from build123d import *

# Parameters (mm, degrees)
BOSS_EXTRUDE1_DEPTH      = 40
CHAMFER1_SIZE            = 25
SKETCH3_W                = 55
SKETCH3_H                = 30.849850196
CUT_EXTRUDE2_DEPTH       = 3
SKETCH5_R                = 1.75
CUT_EXTRUDE4_DEPTH       = 56.226805086
CUT_EXTRUDE3_DEPTH       = 38
SKETCH6_R                = 5.5
SKETCH6_R_2              = 3
BOSS_EXTRUDE2_DEPTH      = 5
CUT_EXTRUDE5_START       = -2
SKETCH7_R                = 3
CUT_EXTRUDE5_DEPTH       = 2
SKETCH9_R                = 3.75
CUT_EXTRUDE7_DEPTH       = 24
SKETCH10_W               = 80.05733418
SKETCH10_H               = 23.210803027
CUT_EXTRUDE8_DEPTH       = 27
BOSS_EXTRUDE3_REACH      = 57.227
BOSS_EXTRUDE3_END_RADIUS = 5.5
SKETCH13_W               = 5
SKETCH13_H               = 8
SKETCH14_W               = 8.301356979
SKETCH14_H               = 17.411858477
CUT_EXTRUDE9_DEPTH       = 38
SKETCH15_W               = 30
SKETCH15_H               = 2
BOSS_EXTRUDE4_DEPTH      = 10


with BuildPart() as part:
    # Sketch1 → Boss-Extrude1 (new body)
    with BuildSketch(Plane.XY):
        Polygon((-27.5, 0), (27.5, 0), (27.5, -15), (35, -10), (35, 0), (27.5, 10), (-27.5, 10), (-35, 0), (-35, -10), (-27.5, -15), align=None)
    extrude(amount=BOSS_EXTRUDE1_DEPTH)

    # Chamfer1
    # the kernel refuses this chamfer: 25 mm, written as the material it takes off along each edge
    with BuildSketch(Plane(origin=(35, -74.292074699, 40), x_dir=(0.027495876610586317, 0, -0.9996219169112966), z_dir=(0, 1, 0)), Plane(origin=(-35, 64.292074699, 40), x_dir=(-0.027495876610586317, 0, -0.9996219169112966), z_dir=(0, -1, 0))) as chamfer1_piece_1:
        Polygon((CHAMFER1_SIZE * 0.999621916911, CHAMFER1_SIZE * 0.0274958766106), (-CHAMFER1_SIZE * 0.0274958766106, CHAMFER1_SIZE * 0.999621916911), (0, 0), align=None)
    extrude(amount=138.584149398, mode=Mode.SUBTRACT)

    # Sketch3 → Cut-Extrude2 (cut)
    with BuildSketch(Plane(origin=(0, 0, 0), x_dir=(-1, 0, 0), z_dir=(0, 0, -1))):
        Rectangle(SKETCH3_W, SKETCH3_H)
    extrude(amount=-CUT_EXTRUDE2_DEPTH, mode=Mode.SUBTRACT)

    # Sketch5 → Cut-Extrude4 (cut, through all)
    with BuildSketch(Plane(origin=(0, 0, 0), x_dir=(-1, 0, 0), z_dir=(0, 0, -1))):
        with Locations(Location((-23, 5, 0), (0, 0, 180))):
            Circle(SKETCH5_R)
        with Locations((23, 5)):
            Circle(SKETCH5_R)
    extrude(amount=-CUT_EXTRUDE4_DEPTH, mode=Mode.SUBTRACT)

    # Sketch4 → Cut-Extrude3 (cut)
    with BuildSketch(Plane.XY.offset(40)):
        Polygon((-34, 1.333333333), (-28.5, 8.666666667), (-28.5, -13.131482908), (-34, -9.464816242), align=None)
    cut_extrude3 = extrude(amount=-CUT_EXTRUDE3_DEPTH, mode=Mode.SUBTRACT)

    # Sketch6 → Boss-Extrude2 (add)
    with BuildSketch(Plane(origin=(-27.5, 0, 0), x_dir=(0, 0, -1), z_dir=(1, 0, 0))):
        with Locations(Location((-7, -9, 0), (0, 0, 180))):
            Circle(SKETCH6_R)
        with Locations((-7, -9)):
            Circle(SKETCH6_R_2, mode=Mode.SUBTRACT)
    boss_extrude2 = extrude(amount=BOSS_EXTRUDE2_DEPTH)

    # Sketch7 → Cut-Extrude5 (cut)
    with BuildSketch(Plane(origin=(-27.5, 0, 0), x_dir=(0, 0, -1), z_dir=(1, 0, 0)).offset(CUT_EXTRUDE5_START)):
        with Locations((-7, -9)):
            Circle(SKETCH7_R)
    cut_extrude5 = extrude(amount=CUT_EXTRUDE5_DEPTH, mode=Mode.SUBTRACT)

    # Mirror1: Cut-Extrude3, Boss-Extrude2, Cut-Extrude5 across plane
    add(cut_extrude3.mirror(Plane(origin=(0, 0, 0), x_dir=(0, 0, 1), z_dir=(1, 0, 0))), mode=Mode.SUBTRACT)
    add(boss_extrude2.mirror(Plane(origin=(0, 0, 0), x_dir=(0, 0, 1), z_dir=(1, 0, 0))))
    add(cut_extrude5.mirror(Plane(origin=(0, 0, 0), x_dir=(0, 0, 1), z_dir=(1, 0, 0))), mode=Mode.SUBTRACT)

    # Sketch9 → Cut-Extrude7 (cut)
    with BuildSketch(Plane.XY.offset(40)):
        with Locations((-23, 5)):
            Circle(SKETCH9_R)
        with Locations((23, 5)):
            Circle(SKETCH9_R)
    extrude(amount=-CUT_EXTRUDE7_DEPTH, mode=Mode.SUBTRACT)

    # Sketch10 → Cut-Extrude8 (cut)
    with BuildSketch(Plane.XY.offset(40)):
        with Locations((1.832814427, -11.605401514)):
            Rectangle(SKETCH10_W, SKETCH10_H)
    extrude(amount=-CUT_EXTRUDE8_DEPTH, mode=Mode.SUBTRACT)

    # Cut-Sweep1: sweep along a path in Sketch11
    with BuildLine(Plane(origin=(0, 0, 0), x_dir=(0, 0, -1), z_dir=(1, 0, 0))) as cut_sweep1_path:
        Line((0, 0), (-9.226976352, 25.350909176))
    # Sketch2 → Cut-Sweep1 (sweep, cut)
    with BuildSketch(Plane.XZ):
        with BuildLine():
            Line((-15, -35), (15, -35))
            Line((15, -35), (15, 25))
            ThreePointArc((15, 25), (12.071067812, 32.071067812), (5, 35))
            Line((5, 35), (-5, 35))
            ThreePointArc((-5, 35), (-12.071067812, 32.071067812), (-15, 25))
            Line((-15, 25), (-15, -35))
        make_face()
    sweep(path=cut_sweep1_path.line, mode=Mode.SUBTRACT)

    # Boss-Extrude3: up to this cylinder (the profile starts outside it)
    boss_extrude3_end = Plane(origin=(-25, -9, 7), z_dir=(-1, 0, 0)) * Cylinder(BOSS_EXTRUDE3_END_RADIUS, 126.454, mode=Mode.PRIVATE)
    # Sketch13 → Boss-Extrude3 (add, up to the surface)
    with BuildSketch(Plane.XZ, mode=Mode.PRIVATE) as boss_extrude3_sk1:
        with Locations((-25, 7)):
            Rectangle(SKETCH13_W, SKETCH13_H)
    boss_extrude3_tool1 = extrude(boss_extrude3_sk1.sketch, amount=BOSS_EXTRUDE3_REACH, mode=Mode.PRIVATE) - boss_extrude3_end
    add(boss_extrude3_tool1.solids().sort_by_distance((-25, 0, 7))[0])

    # Sketch14 → Cut-Extrude9 (cut)
    with BuildSketch(Plane.XY.offset(40)):
        with Locations((-38.15067849, -0.758887004)):
            Rectangle(SKETCH14_W, SKETCH14_H)
    extrude(amount=-CUT_EXTRUDE9_DEPTH, mode=Mode.SUBTRACT)

    # Sketch15 → Boss-Extrude4 (add)
    with BuildSketch(Plane(origin=(0, 10, 0), x_dir=(1, 0, 0), z_dir=(0, 1, 0))):
        with Locations((0, -4)):
            Rectangle(SKETCH15_W, SKETCH15_H)
    extrude(amount=-BOSS_EXTRUDE4_DEPTH)


solid = part.part
Source: CAD feature listing. Evaluate the final solid. Frame: model axes, mm. A direction names the side the tool comes from. Coordinates: 2 decimals unless noted, no trailing zeros. Loops run counter-clockwise (first coordinate to the right, second up) from the corner with the lowest first, then second, coordinate; pieces in that order, holes last. Notation, with made-up numbers: (-25.5, 84) - (26.5, 84) arc R8 cw to (26.5, 94) - close; hole circle Ø2 at (-16.75, 4.5). An arc over 180 degrees is marked (long way). One line per item, written item: value. Start each with the question number.
1. Set-up query: faces 1 (the cylindrical face through (19.254, 5.165, 21.901)), 2 (the flat face through (0, 4, 3)), 3 (the cylindrical face through (25.54, -8.1, 4.14)), 4 (the flat face through (31.212, -11.324, 7.577)). Return all of +Z, -Z, +X, -X, +Y, -Y with unobstructed straight access to the full face (end or side cutting, diameter ignored); none if empty.
2. Section A-A (z = 7). State how many separate pieces and enclosed holes the cut face has, and give its area (3 significant figures).
3. Section C-C (x = -17). Return the cut outline in (y, z).
4. Contact query for flat-ended pins moving along their axis: P1, Ø6, axis at x = 23, y = 5, coming from the -Z side; P2, Ø4, axis at y = 3.5, z = 33.5, coming from the -X side; P3, Ø3, axis at y = 4.5, z = 14.5, coming from the +X side; P4, Ø9, axis at y = -7, z = 4.5, coming from the -X side. Output: stop coordinate, or through.
5. Ray query, L1, parallel to X at y = 5, z = 19.5; L2, parallel to Y at x = 25.1, z = 7; L3, parallel to Z at x = 26.5, y = -9.25. Return the intervals inside material, ascending.
6. Mould query, pull axis Y, two halves, no side actions, for faces 5 (the flat face through (-25, -3, 11)), 6 (the flat face through (-0.4, 10, 4.8)), 7 (the flat face through (-22.5, -5.5, 6.9)). Classes: pulls with the +Y half, pulls with the -Y half, needs draft (parallel to the pull), parting line crosses it, or undercut.
Verdict:
1. face 1: +Z
1. face 2: -Z, +Y
1. face 3: none
1. face 4: +Z, +Y
2. separate pieces: 4
2. enclosed holes: 2
2. area: 359 mm2
3. outline: (0, 3) - (10, 3) - (10, 33) - (0, 33) - close
4. P1: stops at z = 3
4. P2: stops at x = -18.5
4. P3: stops at x = 28.5
4. P4: stops at x = -35
5. L1: x = -28.5 to -26.75, -19.25 to -15, 15 to 19.25, 26.75 to 28.5
5. L2: y = -14.5 to -12, -6 to -3.5, 0 to 10
5. L3: z = 1.51 to 4.01, 9.99 to 12.49
6. face 5: undercut
6. face 6: pulls with the +Y half
6. face 7: needs draft
